```python
from build123d import *

# Parameters (mm, degrees)
F0_W     = 22.8
F0_H     = 28.5
F1_DEPTH = 12.2
F2_R     = 4.930389
F3_DEPTH = 3
F4_R     = 2.022954
F4_R_2   = 0.744862
F5_DEPTH = 3


with BuildPart() as f1:
    # F0 (on Front) → F1 (new body)
    with BuildSketch(Plane.XZ):
        with Locations((11.4, 14.25)):
            Rectangle(F0_W, F0_H)
    extrude(amount=F1_DEPTH)

    # F2 (on face) → F3 (join)
    with BuildSketch(Plane.XY.offset(28.5)):
        with Locations((5.2, -6.1)):
            Circle(F2_R)
    extrude(amount=F3_DEPTH)

    # F4 (on face) → F5 (join)
    with BuildSketch(Plane.XY.offset(31.5)):
        with Locations((5.2, -6.1)):
            Circle(F4_R)
        with Locations((5.2, -6.1)):
            Circle(F4_R_2, mode=Mode.SUBTRACT)
    extrude(amount=F5_DEPTH)


solid = f1.part
```
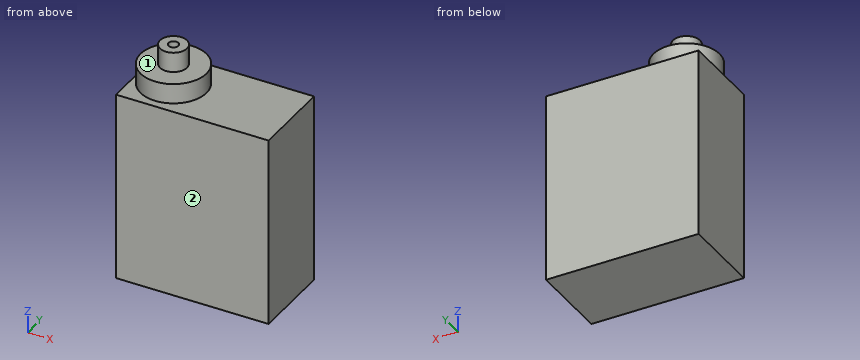
Here's how the part is built. I have some questions about the finished solid (model axes, mm). Face numbers are marked on the shaded views. A direction names the side the tool comes from. Give positions to 0.01 mm unless a question says otherwise; leave off trailing zeros. Order: outer loops, then holes, each group sorted by start corner. A loop starts at its lowest first (then second) coordinate and runs counter-clockwise, first axis right, second up. Notation, with made-up numbers: (42.5, 66) -> (94.5, 66) arc R28 cw to (94.5, 84) -> close; hole circle Ø10 at (13, 80.5). An arc over 180 degrees is marked (long way). Use CSV: the item, a comma, the result in double quotes. Start each with the question number.
Item 1: Suppose I cut it at D-D (y = -9.5). List the corners of the cut face in (x, z) for me.
Item 2: Suppose I cut it at A-A (y = -6.1). List the corners of the cut face in (x, z) for me.
Item 3: On a 3-axis mill with a long thin cutter (end or side, diameter ignored), from which of +Z, -Z, +X, -X, +Y, -Y can I reach the whole of each face in a straight line? I mean the marked faces 1 and 2. Say none if no direction works.
Item 4: Suppose I cut it at C-C (x = 8.25). List the corners of the cut face in (y, z) for me, and give its area (3 significant figures).
Item 5: If I drill on probe 1 along Y at (x, z) = (5.2, 33.7); probe 2 along Z at (x, y) = (14, -9.5); probe 3 along Z at (x, y) = (1.5, -5.75), over which ranges is the centre line in solid material (lowest first)? Write a range as [from, to].
Item 6: I'm going to push flat-ended pins straight in: P1, Ø3.5, axis at x = 8, y = -9, coming from the +Z side; P2, Ø1.6, axis at x = 5.5, y = -6.5, coming from the +Z side; P3, Ø2, axis at x = 12, y = -4, coming from the +Z side. Where does each tip first touch, or does it pass through?
Item 7: Suppose I cut it at B-B (x = 5.2). List the corners of the cut face in (y, z) for me.
Answer block:
1,outline,"(0, 0) -> (22.8, 0) -> (22.8, 28.5) -> (8.77, 28.5) -> (8.77, 31.5) -> (1.63, 31.5) -> (1.63, 28.5) -> (0, 28.5) -> close"
2,outline,"(0, 0) -> (22.8, 0) -> (22.8, 28.5) -> (10.13, 28.5) -> (10.13, 31.5) -> (7.22, 31.5) -> (7.22, 34.5) -> (5.94, 34.5) -> (5.94, 31.5) -> (4.46, 31.5) -> (4.46, 34.5) -> (3.18, 34.5) -> (3.18, 31.5) -> (0.27, 31.5) -> (0.27, 28.5) -> (0, 28.5) -> close"
3,face 1,"+Z"
3,face 2,"+Z, -Z, +X, -X, -Y"
4,outline,"(-12.2, 0) -> (0, 0) -> (0, 28.5) -> (-2.23, 28.5) -> (-2.23, 31.5) -> (-9.97, 31.5) -> (-9.97, 28.5) -> (-12.2, 28.5) -> close"
4,area,"371 mm^2"
5,probe 1,"y = [-8.12, -6.84], [-5.36, -4.08]"
5,probe 2,"z = [0, 28.5]"
5,probe 3,"z = [0, 31.5]"
6,P1,"stops at z = 31.5"
6,P2,"stops at z = 34.5"
6,P3,"stops at z = 28.5"
7,outline,"(-12.2, 0) -> (0, 0) -> (0, 28.5) -> (-1.17, 28.5) -> (-1.17, 31.5) -> (-4.08, 31.5) -> (-4.08, 34.5) -> (-5.36, 34.5) -> (-5.36, 31.5) -> (-6.84, 31.5) -> (-6.84, 34.5) -> (-8.12, 34.5) -> (-8.12, 31.5) -> (-11.03, 31.5) -> (-11.03, 28.5) -> (-12.2, 28.5) -> close"
